Part model, mm, in its own coordinate system. Face numbers are marked on the shaded views. Coordinates: 2 decimals unless noted, no trailing zeros. Order: outer loops, then holes, each group sorted by start corner. A loop starts at its lowest first (then second) coordinate and runs counter-clockwise, first axis right, second up.
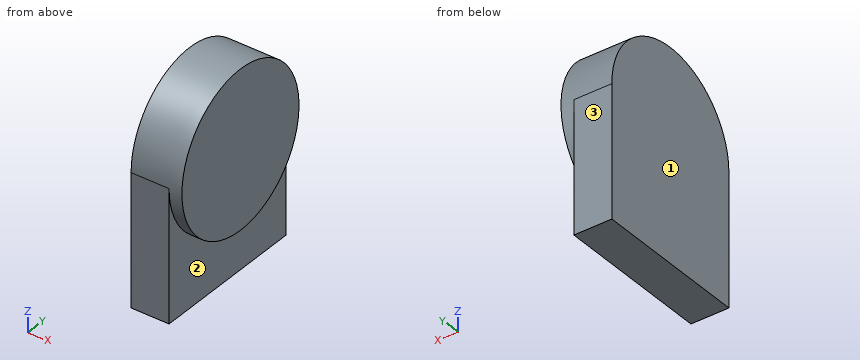
from build123d import *

# Parameters (mm, degrees)
BOSS_EXTRUDE1_DEPTH = 75
SKETCH2_R           = 155
BOSS_EXTRUDE2_DEPTH = 25.4


with BuildPart() as part:
    # Sketch1 → Boss-Extrude1 (new body)
    with BuildSketch(Plane.YZ):
        with BuildLine():
            Line((-155, 0), (-155, -260))
            Line((-155, -260), (155, -260))
            Line((155, -260), (155, 0))
            ThreePointArc((155, 0), (0, 155), (-155, 0))
        make_face()
    extrude(amount=BOSS_EXTRUDE1_DEPTH)

    # Sketch2 → Boss-Extrude2 (add)
    with BuildSketch(Plane(origin=(75, 0, 0), x_dir=(0, 0, -1), z_dir=(1, 0, 0))):
        with Locations(Location((0, 0, 0), (0, 0, 270))):
            Circle(SKETCH2_R)
    extrude(amount=BOSS_EXTRUDE2_DEPTH)


solid = part.part
Q1. Cut at A-A on z = -131. Write the cut outline in (x, y).
Results list:
outline: (0, -155) - (75, -155) - (75, -82.85) - (100.4, -82.85) - (100.4, 82.85) - (75, 82.85) - (75, 155) - (0, 155) - close
Q2. Wall check: line 1 along X through (y, z) = (-11.5, -191); line 2 along Y through (x, z) = (57.5, 26); line 3 along Z through (x, y) = (18, -94.5). Give the ranges that are in metal, low to high.
Results list:
line 1: x = 0 to 75
line 2: y = -152.8 to 152.8
line 3: z = -260 to 122.86
Q3. Mould opens along X. For the marked faces 1, 2 and 3 say: pulls with the +X half, pulls with the -X half, needs draft (parallel to the pull), parting line crosses it, or undercut.
Results list:
face 1: pulls with the -X half
face 2: pulls with the +X half
face 3: needs draft
Q4. Pin check, flat tips, straight feed: pin 1 Ø3 at (x, z) = (10.5, 88.5) entering from -Y; pin 2 Ø4 at (x, z) = (77.5, -191.5) entering from +Y. Stop position of each tip, or through.
Results list:
pin 1: stops at y = -128.28
pin 2: passes through
Q5. Cut at B-B on x = 16. Write the cut outline in (y, z).
Results list:
outline: (-155, -260) - (155, -260) - (155, 0) arc R155 ccw to (-155, 0) - close
